```python
from build123d import *

# Parameters (mm, degrees)
SKETCH_1_R           = 12.5
SKETCH_1_R_2         = 12
EXTRUDE_1_DEPTH      = 40
EXTRUDE_2_DEPTH      = 7
EXTRUDE_2_DEPTH_BACK = 1.034218613
SKETCH_2_R           = 17.5
SKETCH_2_R_2         = 12
SKETCH_3_R           = 17.5
EXTRUDE_3_DEPTH      = 1
SKETCH_4_R           = 12
CUT_EXTRUDE_1_DEPTH  = 1


with BuildPart() as part:
    # Эскиз1 → Бобышка-Вытянуть1 (new body)
    with BuildSketch(Plane.XY):
        Circle(SKETCH_1_R)
        Circle(SKETCH_1_R_2, mode=Mode.SUBTRACT)
    extrude(amount=EXTRUDE_1_DEPTH)

    # Эскиз2 → Бобышка-Вытянуть2 (add, two sides: drawn at the far end of the back side and taken through both)
    with BuildSketch(Plane.XY.offset(40).offset(-EXTRUDE_2_DEPTH_BACK)):
        Circle(SKETCH_2_R)
        Circle(SKETCH_2_R_2, mode=Mode.SUBTRACT)
    extrude(amount=EXTRUDE_2_DEPTH + EXTRUDE_2_DEPTH_BACK)

    # Эскиз3 → Бобышка-Вытянуть3 (add)
    with BuildSketch(Plane(origin=(0, 0, 38.965781387), x_dir=(-1, 0, 0), z_dir=(0, 0, -1))):
        with Locations(Location((0, 0, 0), (0, 0, 180))):
            Circle(SKETCH_3_R)
    extrude(amount=EXTRUDE_3_DEPTH)

    # Эскиз4 → Вырез-Вытянуть1 (cut)
    with BuildSketch(Plane(origin=(0, 0, 37.965781387), x_dir=(-1, 0, 0), z_dir=(0, 0, -1))):
        with Locations(Location((0, 0, 0), (0, 0, 180))):
            Circle(SKETCH_4_R)
    extrude(amount=-CUT_EXTRUDE_1_DEPTH, mode=Mode.SUBTRACT)


solid = part.part
```
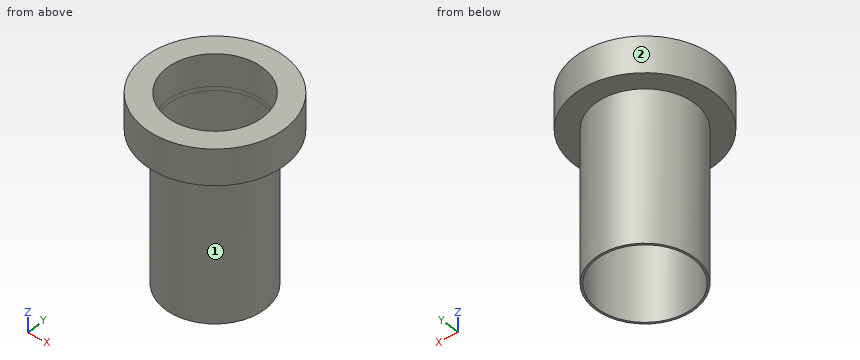
The listing builds one solid part. Answer for the finished solid, in the listing's coordinates (mm). Face numbers are marked on the shaded views. A direction names the side the tool comes from. Round coordinates to 2 decimals unless told otherwise and drop trailing zeros. Loops run counter-clockwise (first coordinate to the right, second up) from the corner with the lowest first, then second, coordinate; pieces in that order, holes last.
1) Given P1, Ø1, axis at x = -4, z = 10.5, coming from the +Y side; P2, Ø1, axis at y = 6.5, z = 7, coming from the -X side; P3, Ø10, axis at x = -8.5, z = 17, coming from the -Y side, each flat-ended and moving along its own axis, determine where each tip first touches the part or whether it passes through.
Outcome:
P1: stops at y = 12
P2: stops at x = -10.97
P3: stops at y = -12
2) A cutting plane is placed at C-C on z = 12. Determine the outline of the cut face in (x, y), plus the area to 3 significant figures.
Outcome:
outline: circle Ø25 at (0, 0); hole circle Ø24 at (0, 0)
area: 38.5 mm2
3) For the marked faces 1 and 2, determine the directions among +Z, -Z, +X, -X, +Y, -Y from which every point of the face is accessible in a straight line to the end or side of a thin tool.
Outcome:
face 1: -Z
face 2: +Z, -Z
4) A cutting plane is placed at A-A on y = 0. Determine the outline of the cut face in (x, z).
Outcome:
outline: (-17.5, 37.97) - (-12.5, 37.97) - (-12.5, 0) - (-12, 0) - (-12, 47) - (-17.5, 47) - close; (12, 0) - (12.5, 0) - (12.5, 37.97) - (17.5, 37.97) - (17.5, 47) - (12, 47) - close
5) A cutting plane is placed at D-D on y = 13.5. Determine the outline of the cut face in (x, z).
Outcome:
outline: (-11.14, 37.97) - (11.14, 37.97) - (11.14, 47) - (-11.14, 47) - close
6) Consider line 1 (X direction, y = 0, z = 12.5); line 2 (X direction, y = 0, z = 43). Determine where each line is inside the solid, lowest interval first.
Outcome:
line 1: x = -12.5 to -12, 12 to 12.5
line 2: x = -17.5 to -12, 12 to 17.5
